The listing builds one solid part. Answer for the finished solid, in the listing's coordinates (mm). A direction names the side the tool comes from. Round coordinates to 2 decimals unless told otherwise and drop trailing zeros. Loops run counter-clockwise (first coordinate to the right, second up) from the corner with the lowest first, then second, coordinate; pieces in that order, holes last. Notation, with made-up numbers: (63, 73) -> (101, 73) arc R17 cw to (101, 101) -> close; hole circle Ø1 at (58, -29). An arc over 180 degrees is marked (long way). Use a Markdown table: item, result. Add a question column.
Q1. For a pull along Y with two mould halves and no side action, classify faces 1 (the flat face through (5, 14, 2)), 2 (the flat face through (6, 0, 0)), 3 (the cylindrical face through (2.23, -4.81, 2.54)) as released by +Y, released by -Y, zero draft, split by the parting line, or undercut.
Q2. Section C-C on x = 5.5 is taken. Give the vertices of the cut face in (y, z), then the cut area to 3 significant figures.
Q3. Which of the six approach directions +Z, -Z, +X, -X, +Y, -Y give full straight-line access (tool end or side, diameter ignored) to faces 4 (the cylindrical face through (2.22, 4.83, 2.54)), 5 (the cylindrical face through (2.6, 13.43, 2.54))?
Q4. Section A-A on z = 3.05 is taken. Give the vertices of the cut face in (x, y), then the cut area to 3 significant figures.
Q5. Given pin 1 Ø2.5 at (x, y) = (6, 10) entering from +Z; pin 2 Ø2 at (x, y) = (4.5, -4.5) entering from -Z, each flat-ended and moving along its own axis, determine where each tip first touches the part or whether it passes through.
Q6. Section D-D on y = 1 is taken. Give the vertices of the cut face in (x, z), then the cut area to 3 significant figures.
Q7. Section B-B on y = -9.5 is taken. Give the vertices of the cut face in (x, z), then the cut area to 3 significant figures.
Q8. Consider line 1 (Y direction, x = 6.5, z = 2.6); line 2 (X direction, y = -10.25, z = 0.6); line 3 (X direction, y = 9.5, z = 3.95). Determine where each line is inside the solid, lowest interval first.
from build123d import *

# Parameters (mm, degrees)
ESQUISSE1_R        = 1.5
BOSS_EXTRU_1_DEPTH = 5
CONG_1_R           = 5
CONG_2_R           = 2


with BuildPart() as part:
    # Esquisse1 → Boss.-Extru.1 (new body)
    with BuildSketch(Plane.XY):
        with BuildLine():
            Line((2, 14), (2, 4.582575695))
            ThreePointArc((2, 4.582575695), (5, 0), (2, -4.582575695))
            Line((2, -4.582575695), (2, -14))
            Line((2, -14), (11, -14))
            Line((11, -14), (11, 14))
            Line((11, 14), (2, 14))
        make_face()
        with Locations((6, 10)):
            Circle(ESQUISSE1_R, mode=Mode.SUBTRACT)
        with Locations(Location((6, -10, 0), (0, 0, 180))):
            Circle(ESQUISSE1_R, mode=Mode.SUBTRACT)
    extrude(amount=BOSS_EXTRU_1_DEPTH)

    # Congé1
    cong_1_edges = [part.edges().sort_by_distance(p)[0] for p in [
        (11, 14, 2.5),
        (11, -14, 2.5),
    ]]
    fillet(cong_1_edges, radius=CONG_1_R)

    # Congé2
    cong_2_edges = [part.edges().sort_by_distance(p)[0] for p in [
        (2, -14, 2.5),
        (2, -4.582575695, 2.5),
        (2, 4.582575695, 2.5),
        (2, 14, 2.5),
    ]]
    fillet(cong_2_edges, radius=CONG_2_R)


solid = part.part
Checked values:
| question | item | result |
|---|---|---|
| 1 | face 1 | released by +Y |
| 1 | face 2 | zero draft |
| 1 | face 3 | undercut |
| 2 | outline | (-14, 0) -> (-11.41, 0) -> (-11.41, 5) -> (-14, 5) -> close; (-8.59, 0) -> (8.59, 0) -> (8.59, 5) -> (-8.59, 5) -> close; (11.41, 0) -> (14, 0) -> (14, 5) -> (11.41, 5) -> close |
| 2 | area | 112 mm2 |
| 3 | face 4 | +Z, -Z, -X |
| 3 | face 5 | +Z, -Z, -X, +Y |
| 4 | outline | (2, -12) arc R2 ccw to (4, -14) -> (6, -14) arc R5 ccw to (11, -9) -> (11, 9) arc R5 ccw to (6, 14) -> (4, 14) arc R2 ccw to (2, 12) -> (2, 5.74) arc R2 ccw to (2.86, 4.1) arc R5 cw to (2.86, -4.1) arc R2 ccw to (2, -5.74) -> close; hole circle Ø3 at (6, -10); hole circle Ø3 at (6, 10) |
| 4 | area | 205 mm2 |
| 5 | pin 1 | passes through |
| 5 | pin 2 | stops at z = 0 |
| 6 | outline | (4.9, 0) -> (11, 0) -> (11, 5) -> (4.9, 5) -> close |
| 6 | area | 30.5 mm2 |
| 7 | outline | (2, 0) -> (4.59, 0) -> (4.59, 5) -> (2, 5) -> close; (7.41, 0) -> (10.97, 0) -> (10.97, 5) -> (7.41, 5) -> close |
| 7 | area | 30.7 mm2 |
| 8 | line 1 | y = -13.97 to -11.41, -8.59 to 8.59, 11.41 to 13.97 |
| 8 | line 2 | x = 2 to 4.52, 7.48 to 10.84 |
| 8 | line 3 | x = 2 to 4.59, 7.41 to 10.97 |
